Autodesk Inventor part; units mm, degrees
ref_plane "YZ Plane" through (0, 0, 0) normal (1, 0, 0) x (0, 1, 0)
ref_plane "XZ Plane" through (0, 0, 0) normal (0, 1, 0) x (-1, 0, 0)
ref_plane "XY Plane" through (0, 0, 0) normal (0, 0, 1) x (1, 0, 0)
sketch "スケッチ1" plane through (0, 0, 0) normal (0, 0, 1) x (1, 0, 0)
  line L0 (-18, -8) -> (18, -8) construction
  line L1 (18, -8) -> (18, 8) construction
  line L2 (18, 8) -> (-18, 8) construction
  line L3 (-18, 8) -> (-18, -8) construction
  line L4 (-18, -8) -> (18, 8) construction
  line L5 (18, -8) -> (-18, 8) construction
  circle A0 centre (-18, 8) radius 1.1
  circle A1 centre (18, 8) radius 1.1
  circle A2 centre (-18, -8) radius 1.1
  circle A3 centre (18, -8) radius 1.1
  circle A4 centre (-18, 8) radius 2
  circle A5 centre (-18, -8) radius 2
  line L6 (-16, 8) -> (-16, -8)
  circle A6 centre (-35.2333, 5) radius 2.25
  circle A7 centre (-35.2333, 5) radius 3.5
  line L7 (-35.5357, 8.4869) -> (-18.1728, 9.9925)
  line L8 (-37.1418, 2.0661) -> (-19.0906, -9.6765)
  circle A8 centre (11.5, 0) radius 8
  line L9 (-35.2333, 5) -> (11.5, 0) construction
  point P0 (0, 0)
  point P1 (-16, 0)
  dimension "d0" = 36
  dimension "d1" = 16
  dimension "d2" = 2.2
  dimension "d5" = 36
  dimension "d8" = 16
  dimension "d11" = 4
  dimension "d12" = 4
  dimension "d13" = 4.5
  dimension "d14" = 7
  dimension "d16" = 5
  dimension "d19" = 47
extrude "押し出し1" add sketch "スケッチ1" along normal blind 1.5 contours A4 | L6 A5 L8 A7 L7 A4 | A5 | A7
sketch "スケッチ2" plane through (0, 0, 0) normal (0, 0, -1) x (-1, 0, 0)
  line L0 (37.1418, 2.0661) -> (19.0906, -9.6765)
  arc A0 (37.1418, 2.0661) -> (35.5357, 8.4869) centre (35.2333, 5) ccw
  line L1 (18.1728, 9.9925) -> (35.5357, 8.4869)
  arc A1 (18.1728, 9.9925) -> (16, 8) centre (18, 8) ccw
  line L2 (16, -8) -> (16, 8)
  arc A2 (16, -8) -> (19.0906, -9.6765) centre (18, -8) ccw
  circle A3 centre (18, -8) radius 1.1
  circle A4 centre (18, 8) radius 1.1
  circle A5 centre (35.2333, 5) radius 2.25
  line L3 (18, -8) -> (36.0512, 3.7426)
  arc A6 (36.0512, 3.7426) -> (35.3629, 6.4944) centre (35.2333, 5) ccw
  line L4 (35.3629, 6.4944) -> (18, 8)
  line L5 (18, 8) -> (18, -8)
  circle A7 centre (18, 8) radius 2
  circle A8 centre (18, -8) radius 2
  circle A9 centre (35.2333, 5) radius 3.5
  point P0 (0, 0)
  point P1 (33.4005, 2.0183)
  point P2 (32.2124, 6.7676)
  point P3 (19.9925, 7.8272)
  point P4 (18, 6)
  point P5 (33.6921, 6.6393)
  point P6 (34.6454, 2.8281)
  point P7 (20, 7.9971)
  point P8 (18.4708, 6.0562)
  point P9 (19, 2.9103)
  point P10 (18, -6.9)
  point P11 (18.9221, -7.4002)
  point P12 (18, -6)
  point P13 (19.6765, -6.9094)
  point P14 (18, 6.9)
  point P15 (19.0959, 7.905)
  dimension "d20" = 2
extrude "押し出し2" cut sketch "スケッチ2" against normal through all contours L3 A8 L5 A7 L4 A9 | A5 L4 A6 L3 | L3 L5 A3 | A4 L5 L4 picked at (34.8052, 4.9839) picked at (18.0902, -7.2779) picked at (18.7117, 7.8482)
fillet "フィレット1" radius 2 6 edges at (-33.4005, 2.0183, 0.75) (-32.2124, 6.7676, 0.75) (-18, -6, 0.75) (-19.6765, -6.9094, 0.75) (-18, 6, 0.75) (-19.9925, 7.8272, 0.75)
equation "\"d5\" = d0"
equation "\"d8\" = d1"
properties part number "servolink" material "アルミニウム 2014-T4"
Here's how the part is built. I have some questions about the finished solid (model axes, mm). A direction names the side the tool comes from. Give positions to 0.01 mm unless a question says otherwise; leave off trailing zeros. Order: outer loops, then holes, each group sorted by start corner. A loop starts at its lowest first (then second) coordinate and runs counter-clockwise, first axis right, second up. Notation, with made-up numbers: M 57.5,-17.5 L 98.5,-17.5 A14 ccw 98.5,7.5 Z; hole C 3,83 d10. An arc over 180 degrees is marked long. Answer as a JSON object with one key per item and string values. Group by question number.
1) I'm going to push flat-ended pins straight in: pin 1 Ø6 at (x, y) = (-30, 7) entering from -Z; pin 2 Ø0.8 at (y, z) = (1, 1) entering from -X. Where does each tip first touch, or does it pass through?
2) We'd pull the mould along Y, two halves only. Please class faces 3 (the cylindrical face through (-31.19, 6.345, 0.76)), 4 (the cylindrical face through (-16.665, 9.49, 0.74)), 5 (the flat face through (-29.1, -1.4, 1.5)): pulls with the +Y half, pulls with the -Y half, needs draft (parallel to the pull), parting line crosses it, or undercut.
3) Suppose I cut it at A-A, the plane x = -17.5. Write out the boundary of the cut face in (y, z), plus the area to 3 significant figures.
4) Suppose I cut it at B-B, the plane y = -8.5. Write out the boundary of the cut face in (x, z), plus the area to 3 significant figures.
5) Please list where these lines run through material, in increasing order: L1, parallel to Y at x = -17, z = 0.8; L2, parallel to X at y = 5, z = 0.5; L3, parallel to Y at x = -18.5, z = 1.2. Write a range as [from, to].
6) Suppose I cut it at C-C, the plane x = -34. Write out the boundary of the cut face in (y, z).
7) Suppose I cut it at D-D, the plane z = 0.35. Count the separate pieces of the cut face and the enclosed holes in it, plus the area to 3 significant figures.
8) On a 3-axis mill with a long thin cutter (end or side, diameter ignored), from which of +Z, -Z, +X, -X, +Y, -Y can I reach the whole of each face in a straight line? I mean faces 1 (the flat face through (-18, 0, 1)), 2 (the flat face through (-26.98, 9.23, 0.74)). Say none if no direction works.
Results found:
{
 "1": {"pin 1": "z = 0", "pin 2": "x = -36.12"},
 "2": {"face 3": "undercut", "face 4": "pulls with the +Y half", "face 5": "needs draft"},
 "3": {"outline": "M -9.94,0 L -8.98,0 L -8.98,1.5 L -9.94,1.5 Z; M -7.02,0 L 7.02,0 L 7.02,1.5 L -7.02,1.5 Z; M 8.98,0 L 9.94,0 L 9.94,1.5 L 8.98,1.5 Z", "area": "23.9 mm²"},
 "4": {"outline": "M -20.9,0 L -18.98,0 L -18.98,1.5 L -20.9,1.5 Z; M -17.02,0 L -16.06,0 L -16.06,1.5 L -17.02,1.5 Z", "area": "4.31 mm²"},
 "5": {"L1": "[-9.73, -8.46], [-7.54, 7.54], [8.46, 9.73]", "L2": "[-38.73, -37.48], [-32.98, -31.73], [-18.05, -16]", "L3": "[-9.94, -8.98], [-7.02, -5.64], [5.86, 7.02], [8.98, 9.96]"},
 "6": {"outline": "M 0.02,0 L 3.12,0 L 3.12,1.5 L 0.02,1.5 Z; M 6.88,0 L 8.62,0 L 8.62,1.5 L 6.88,1.5 Z"},
 "7": {"separate pieces": "1", "enclosed holes": "4", "area": "132 mm²"},
 "8": {"face 1": "+Z, -Z", "face 2": "+Z, -Z, -X, +Y"}
}
